Autodesk Inventor part; units mm, degrees
ref_plane "YZ Plane" through (0, 0, 0) normal (1, 0, 0) x (0, 1, 0)
ref_plane "XZ Plane" through (0, 0, 0) normal (0, 1, 0) x (-1, 0, 0)
ref_plane "XY Plane" through (0, 0, 0) normal (0, 0, 1) x (1, 0, 0)
sketch "Sketch1" plane through (0, 0, 0) normal (0, 0, 1) x (1, 0, 0)
  arc A0 (-21.082, 40.132) -> (21.082, 40.132) centre (0, 40.132) ccw
  line L0 (-21.082, 40.132) -> (-21.082, 0)
  line L1 (21.082, 40.132) -> (21.082, 0)
  line L2 (-21.082, 0) -> (21.082, 0)
  line L3 (-21.082, 0) -> (-27.432, 0)
  line L4 (-27.432, 0) -> (-27.432, 63.5)
  line L5 (-27.432, 63.5) -> (-21.082, 63.5)
  line L6 (-21.082, 63.5) -> (-21.082, 0)
  line L7 (21.082, 0) -> (27.432, 0)
  line L8 (27.432, 0) -> (27.432, 63.5)
  line L9 (27.432, 63.5) -> (21.082, 63.5)
  line L10 (21.082, 63.5) -> (21.082, 0)
  point P0 (0, 0)
  dimension "diameterOfPipe" = 42.164
  dimension "d6" = 6.35
  dimension "d7" = 63.5
  dimension "d8" = 6.35
  dimension "d9" = 63.5
  dimension "d13" = 19.05
revolve "Revolution1" add sketch "Sketch1" angle 360 about axis through (-21.082, 0, 0) along (1, 0, 0)
sketch "Sketch3" plane through (27.432, 0, 0) normal (1, 0, 0) x (0, 0, -1)
  line L0 (7.9189, 0) -> (3.9595, -6.858)
  line L1 (3.9595, -6.858) -> (-3.9595, -6.858)
  line L2 (-3.9595, -6.858) -> (-7.9189, 0)
  line L3 (-7.9189, 0) -> (-3.9595, 6.858)
  line L4 (-3.9595, 6.858) -> (3.9595, 6.858)
  line L5 (3.9595, 6.858) -> (7.9189, 0)
  point P0 (0, 0)
  point P1 (0, 0)
  dimension "hexWidth" = 13.716
extrude "Extrusion2" cut sketch "Sketch3" against normal through all
split "Split1" plane through (0, 0, 0) removes the side toward (-1, 0, 0)
equation "\"d6\" = widthOfOutside"
equation "\"d8\" = widthOfOutside"
equation "\"widthOfOutside\" = 6.35"
properties part number "halfWheelForHangingAndMoving" material "PBT Plastic"
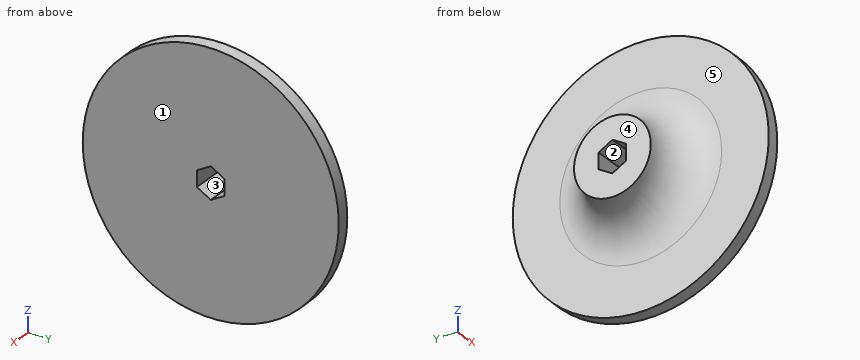
Model file for the job. Use its own axes, mm. Face numbers are marked on the shaded views. A direction names the side the tool comes from. Coordinates: 2 decimals unless noted, no trailing zeros. Order: outer loops, then holes, each group sorted by start corner. A loop starts at its lowest first (then second) coordinate and runs counter-clockwise, first axis right, second up. Notation, with made-up numbers: M -16,43 L 4,43 A18 cw 4,49 Z; hole C 86.25,5 d3. An arc over 180 degrees is marked long. Return JSON: item names as keys, results as strings.
1. Saw through at B-B (x = 13.75). Give the cut face in (y, z).
Ans:
{"outline": "C 0,0 d48.3; hole M -6.86,-3.96 L 0,-7.92 L 6.86,-3.96 L 6.86,3.96 L 0,7.92 L -6.86,3.96 Z"}
2. Drill centre lines: probe 1 along X at (y, z) = (40, 4.5); probe 2 along Y at (x, z) = (9.25, 7); probe 3 along Y at (x, z) = (15.75, 0). Where is each one in solid material? Low to high.
Ans:
{"probe 1": "21.08 to 27.43", "probe 2": "-20 to -1.59, 1.59 to 20", "probe 3": "-26.12 to -6.86, 6.86 to 26.12"}
3. Saw through at C-C (y = 52). Give the cut face in (x, z).
Ans:
{"outline": "M 21.08,-36.45 L 27.43,-36.45 L 27.43,36.45 L 21.08,36.45 Z"}
4. Tool access for the marked faces 3, 4 and 5: list every direction of +Z, -Z, +X, -X, +Y, -Y with a clear straight run to the whole face (end or side of a thin tool).
Ans:
{"face 3": "+X, -X", "face 4": "+Z, -Z, -X, +Y, -Y", "face 5": "-X"}
5. Pull direction Z, two halves, no side cores. Call the marked faces 1 and 2: +Z half, -Z half, draft (parallel to the pull), parting line (faces both ways), or undercut.
Ans:
{"face 1": "draft", "face 2": "undercut"}
6. Flat gauge pins, fed straight in: pin 1 (4 mm diameter, centred on y = 27, z = 42.5, fed in from -X); pin 2 (4 mm diameter, centred on x = 16.5, z = -1, fed in from -Y); pin 3 (3 mm diameter, centred on x = 21.5, z = -33, fed in from +Y). Where does each tip first touch, or does it go through?
Ans:
{"pin 1": "x = 21.08", "pin 2": "y = -30.01", "pin 3": "y = 55.14"}
7. Saw through at D-D (z = 42). Give the cut face in (x, y), and give its area (3 significant figures).
Ans:
{"outline": "M 21.08,-47.63 L 27.43,-47.63 L 27.43,47.63 L 21.08,47.63 Z", "area": "605 mm^2"}
8. Saw through at A-A (z = 0). Give the cut face in (x, y).
Ans:
{"outline": "M 0,-19.05 A21.08 cw 21.08,-40.13 L 21.08,-63.5 L 27.43,-63.5 L 27.43,-6.86 L 0,-6.86 Z; M 0,6.86 L 27.43,6.86 L 27.43,63.5 L 21.08,63.5 L 21.08,40.13 A21.08 cw 0,19.05 Z"}
